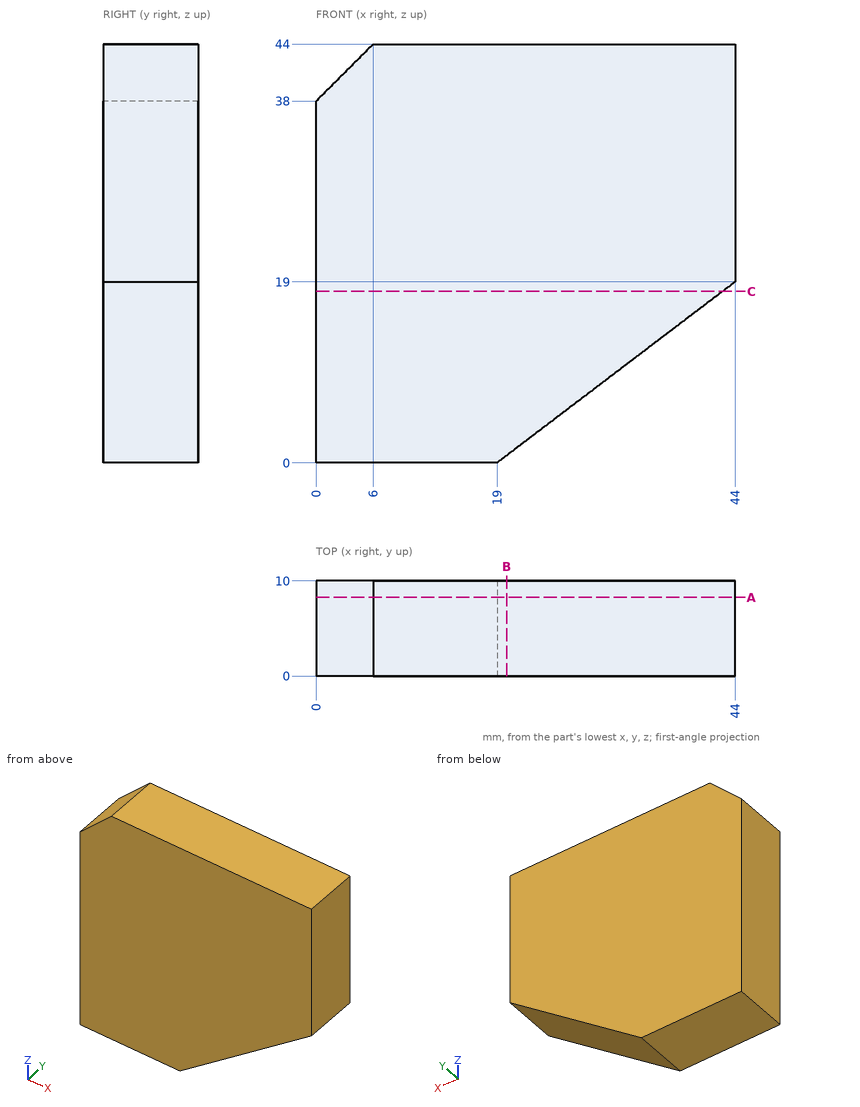
Geometry: see drawing. Coordinates: mm, zero at the bounding-box minimum. Round coordinates to 2 decimals unless told otherwise and drop trailing zeros. Write each loop counter-clockwise with the first axis right and the second up, starting at its lowest first coordinate (ties: lowest second). Pieces come first, ordered by that corner, then holes. Notation, with made-up numbers: (11.25, 15) - (59.25, 15) arc R16 ccw to (59.25, 40) - close; hole circle Ø3 at (-31, -39.75). An arc over 180 degrees is marked (long way). Use CSV: the item, a comma, the result in double quotes. Start each with the question number.
(1) Cut plane A-A, the plane y = 8.25. Return loops of the section in (x, z).
(2) Cut plane B-B, the plane x = 20. Return loops of the section in (y, z).
(3) Material intervals for probe 1 along X at (y, z) = (4.75, 10.5); probe 2 along Z at (x, y) = (40.5, 7.75); probe 3 along Z at (x, y) = (38, 4.25), sorted ascending. Write a range as [from, to].
(4) First-contact query: pin 1 Ø1.5 at (x, y) = (29.5, 2.5) entering from -Z; pin 2 Ø2 at (x, y) = (28.5, 4) entering from -Z. Flat tips, straight axial feed; report the tip coordinate or a pass-through.
(5) Cut plane C-C, the plane z = 18. Return loops of the section in (x, y).
Geometry says:
1,outline,"(0, 0) - (19, 0) - (44, 19) - (44, 44) - (6, 44) - (0, 38) - close"
2,outline,"(0, 0.76) - (10, 0.76) - (10, 44) - (0, 44) - close"
3,probe 1,"[0, 32.82]"
3,probe 2,"[16.34, 44]"
3,probe 3,"[14.44, 44]"
4,pin 1,"z = 7.41"
4,pin 2,"z = 6.46"
5,outline,"(0, 0) - (42.68, 0) - (42.68, 10) - (0, 10) - close"
